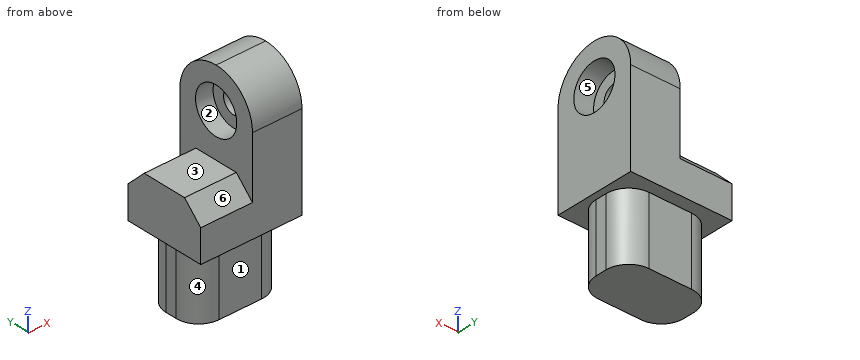
from build123d import *

# Parameters (mm, degrees)
SKETCH2_W                                            = 24.765
SKETCH2_H                                            = 15.875
BOSS_EXTRUDE1_DEPTH                                  = 19.05
SKETCH3_W                                            = 28.575
SKETCH3_H                                            = 22.86
BOSS_EXTRUDE2_DEPTH                                  = 38.1
SKETCH4_W                                            = 14.605
SKETCH4_H                                            = 23.8125
CUT_EXTRUDE1_DEPTH                                   = 47.6725
FILLET5_R                                            = 11.43
FILLET3_R                                            = 6.35
CHAMFER1_SIZE                                        = 5.08
CBORE_FOR_1_4_FILLISTER_HEAD_MACHINE_SCR_D           = 6.35
CBORE_FOR_1_4_FILLISTER_HEAD_MACHINE_SCR_CBORE_D     = 12.954
CBORE_FOR_1_4_FILLISTER_HEAD_MACHINE_SCR_CBORE_DEPTH = 5.588


with BuildPart() as part:
    # Sketch2 → Boss-Extrude1 (new body)
    with BuildSketch(Plane.XY):
        Rectangle(SKETCH2_W, SKETCH2_H)
    extrude(amount=-BOSS_EXTRUDE1_DEPTH)

    # Sketch3 → Boss-Extrude2 (add)
    with BuildSketch(Plane.XY):
        Rectangle(SKETCH3_W, SKETCH3_H)
    extrude(amount=BOSS_EXTRUDE2_DEPTH)

    # Sketch4 → Cut-Extrude1 (cut, through all)
    with BuildSketch(Plane(origin=(0, -11.43, 0), x_dir=(-1, 0, 0), z_dir=(0, -1, 0))):
        with Locations((6.985, -26.19375)):
            Rectangle(SKETCH4_W, SKETCH4_H)
    extrude(amount=-CUT_EXTRUDE1_DEPTH, mode=Mode.SUBTRACT)

    # Fillet5
    fillet5_edges = [part.edges().sort_by_distance(p)[0] for p in [
        (7.3025, -11.43, 38.1),
        (7.3025, 11.43, 38.1),
    ]]
    fillet(fillet5_edges, radius=FILLET5_R - 0.0001)  # a hair under: the kernel refuses the full size

    # Fillet3
    fillet3_edges = [part.edges().sort_by_distance(p)[0] for p in [
        (-12.3825, 7.9375, -9.525),
        (12.3825, 7.9375, -9.525),
        (12.3825, -7.9375, -9.525),
        (-12.3825, -7.9375, -9.525),
    ]]
    fillet(fillet3_edges, radius=FILLET3_R)

    # Chamfer1
    chamfer1_edges = [part.edges().sort_by_distance(p)[0] for p in [
        (-6.985, 11.43, 14.2875),
        (-6.985, -11.43, 14.2875),
    ]]
    chamfer(chamfer1_edges, length=CHAMFER1_SIZE)

    # CBORE for 1/4 Fillister Head Machine Screw1 (through all)
    with Locations(Plane(origin=(14.2875, 0, 26.67), x_dir=(0, 0, 1), z_dir=(1, 0, 0))):
        with Locations((0, 0)):
            cbore_for_1_4_fillister_head_machine_scr = CounterBoreHole(CBORE_FOR_1_4_FILLISTER_HEAD_MACHINE_SCR_D / 2, CBORE_FOR_1_4_FILLISTER_HEAD_MACHINE_SCR_CBORE_D / 2, CBORE_FOR_1_4_FILLISTER_HEAD_MACHINE_SCR_CBORE_DEPTH)

    # Mirror1: CBORE for 1/4 Fillister Head Machine Screw1 across plane
    add(cbore_for_1_4_fillister_head_machine_scr.mirror(Plane(origin=(6.985, 0, 0), x_dir=(0, 0, 1), z_dir=(1, 0, 0))), mode=Mode.SUBTRACT)


solid = part.part
Verification items for the finished model (mm, model axes). Face numbers are marked on the shaded views. A direction names the side the tool comes from. Give positions to 0.01 mm unless a question says otherwise; leave off trailing zeros. Loops run counter-clockwise (first coordinate to the right, second up) from the corner with the lowest first, then second, coordinate; pieces in that order, holes last. Notation, with made-up numbers: (63.5, -7) - (74.5, -7) arc R13 cw to (74.5, 16) - close; hole circle Ø2 at (9.25, 43.5). An arc over 180 degrees is marked (long way). Write item = value, one per line. Start each with the question number.
Q1. Cross-section at D-D, the plane y = -4.25. Enter the section's corners in (x, z), and give its area (3 significant figures).
Q2. Cross-section at C-C, the plane y = 2.5. Enter the section's corners in (x, z), and give its area (3 significant figures).
Q3. Depth check by flat-ended pin: P1, Ø3.5, axis at x = -2.5, z = -9.5, coming from the -Y side; P2, Ø4, axis at y = 0.5, z = 24, coming from the -X side; P3, Ø12, axis at x = 11.5, y = -1.5, coming from the +Z side; P4, Ø1.6, axis at y = -0.5, z = -13, coming from the -X side. Enter the tip coordinate at first touch or a pass-through.
Q4. Mould release check, pull along Y, two halves, no side actions. Record for the marked faces 1, 2 and 3: released by +Y, released by -Y, zero draft, split by the parting line, or undercut.
Q5. Cross-section at B-B, the plane z = -2.5. Enter the section's corners in (x, y).
Q6. Tool access check on the marked faces 4, 5 and 6. Record the directions out of +Z, -Z, +X, -X, +Y, -Y that give a thin tool (end or side, any length) a straight path to the whole face; none if there is none.
Q7. Cross-section at A-A, the plane x = -0.75. Enter the section's corners in (y, z), and give its area (3 significant figures).
Q8. Thickness scan on line 1 (Y direction, x = 7.15, z = 26.67) (3 decimals); line 2 (Z direction, x = -5.5, y = -6); line 3 (X direction, y = 9.5, z = 32). Record the ranges inside material, lowest first.
Answer key:
q1.outline = (-14.29, 0) - (-11.8, 0) - (-11.8, -19.05) - (11.8, -19.05) - (11.8, 0) - (14.29, 0) - (14.29, 21.78) - (8.7, 21.78) - (8.7, 31.56) - (14.29, 31.56) - (14.29, 37.28) - (0.32, 37.28) - (0.32, 31.56) - (5.27, 31.56) - (5.27, 21.78) - (0.32, 21.78) - (0.32, 14.29) - (-14.29, 14.29) - close
q1.area = 1,080 mm^2
q2.outline = (-14.29, 0) - (-12.32, 0) - (-12.32, -19.05) - (12.32, -19.05) - (12.32, 0) - (14.29, 0) - (14.29, 20.69) - (8.7, 20.69) - (8.7, 24.71) - (5.27, 24.71) - (5.27, 20.69) - (0.32, 20.69) - (0.32, 14.29) - (-14.29, 14.29) - close; (0.32, 32.65) - (5.27, 32.65) - (5.27, 28.63) - (8.7, 28.63) - (8.7, 32.65) - (14.29, 32.65) - (14.29, 37.82) - (0.32, 37.82) - close
q2.area = 1,070 mm^2
q3.P1 = -7.94
q3.P2 = 5.27
q3.P3 = 38.1
q3.P4 = -12.38
q4.face_1 = released by -Y
q4.face_2 = undercut
q4.face_3 = zero draft
q5.outline = (-12.38, -1.59) arc R6.35 ccw to (-6.03, -7.94) - (6.03, -7.94) arc R6.35 ccw to (12.38, -1.59) - (12.38, 1.59) arc R6.35 ccw to (6.03, 7.94) - (-6.03, 7.94) arc R6.35 ccw to (-12.38, 1.59) - close
q6.face_4 = -Z, -X, -Y
q6.face_5 = +X
q6.face_6 = +Z, -X, -Y
q7.outline = (-11.43, 0) - (-7.94, 0) - (-7.94, -19.05) - (7.94, -19.05) - (7.94, 0) - (11.43, 0) - (11.43, 9.21) - (6.35, 14.29) - (-6.35, 14.29) - (-11.43, 9.21) - close
q7.area = 603 mm^2
q8.line_1 = -11.43 to -3.175, 3.175 to 11.43
q8.line_2 = -19.05 to 14.29
q8.line_3 = 0.32 to 14.29
